Answer from the drawing. Dimensions are ordinates in mm from the lowest x, y and z of the part. A direction names the side the tool comes from. Coordinates: 2 decimals unless noted, no trailing zeros. Order: outer loops, then holes, each group sorted by start corner. A loop starts at its lowest first (then second) coordinate and runs counter-clockwise, first axis right, second up. Notation, with made-up numbers: (36.25, -7.5) -> (84.25, -7.5) arc R19 cw to (84.25, -0.5) -> close; hole circle Ø10 at (1.5, -24.75). An arc over 180 degrees is marked (long way). Answer in a Markdown table with one row per item.
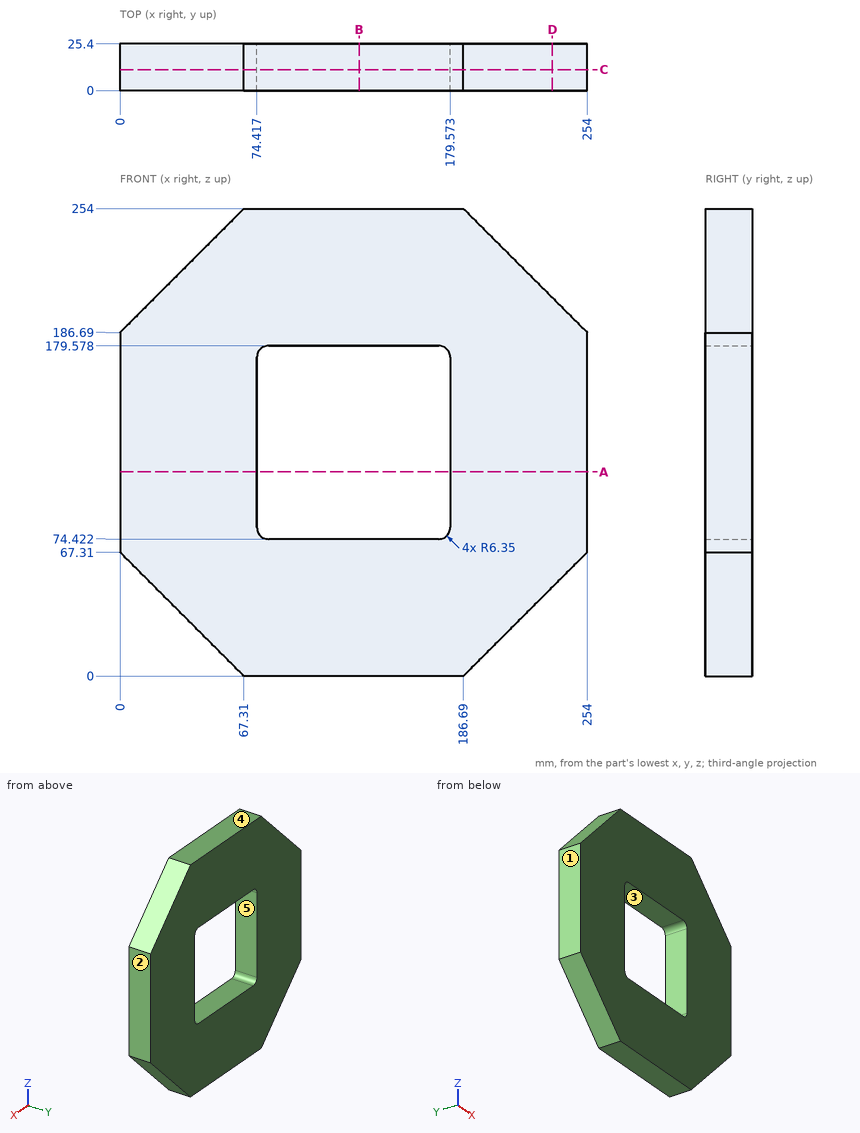
Q1. Consider line 1 (X direction, y = 9.75, z = 133); line 2 (Z direction, x = 122.5, y = 3.5); line 3 (Z direction, x = 177, y = 23). Determine where each line is inside the solid, lowest interval first.
Outcome:
| item | result |
|---|---|
| line 1 | 0 to 74.42, 179.57 to 254 |
| line 2 | 0 to 74.42, 179.58 to 254 |
| line 3 | 0 to 75.67, 178.33 to 254 |
Q2. For the marked faces 4 and 5, determine the directions among +Z, -Z, +X, -X, +Y, -Y from which every point of the face is accessible in a straight line to the end or side of a thin tool.
Outcome:
| item | result |
|---|---|
| face 4 | +Z, +X, -X, +Y, -Y |
| face 5 | +Y, -Y |
Q3. The part is cut by section B-B (x = 130). Write down the section's boundary in (y, z), then the cut area to 3 significant figures.
Outcome:
| item | result |
|---|---|
| outline | (0, 0) -> (25.4, 0) -> (25.4, 74.42) -> (0, 74.42) -> close; (0, 179.58) -> (25.4, 179.58) -> (25.4, 254) -> (0, 254) -> close |
| area | 3,780 mm² |
Q4. The part is cut by section A-A (z = 111). Write down the section's boundary in (x, y).
Outcome:
| item | result |
|---|---|
| outline | (0, 0) -> (74.42, 0) -> (74.42, 25.4) -> (0, 25.4) -> close; (179.57, 0) -> (254, 0) -> (254, 25.4) -> (179.57, 25.4) -> close |
Q5. For a pull along X with two mould halves and no side action, classify the marked faces 1, 2 and 3 as pulls with the +X half, pulls with the -X half, needs draft (parallel to the pull), parting line crosses it, or undercut.
Outcome:
| item | result |
|---|---|
| face 1 | pulls with the -X half |
| face 2 | pulls with the +X half |
| face 3 | undercut |
Q6. The part is cut by section D-D (x = 235). Write down the section's boundary in (y, z), then the cut area to 3 significant figures.
Outcome:
| item | result |
|---|---|
| outline | (0, 48.31) -> (25.4, 48.31) -> (25.4, 205.69) -> (0, 205.69) -> close |
| area | 4,000 mm² |
Q7. The part is cut by section C-C (y = 11.5). Write down the section's boundary in (x, z).
Outcome:
| item | result |
|---|---|
| outline | (0, 67.31) -> (67.31, 0) -> (186.69, 0) -> (254, 67.31) -> (254, 186.69) -> (186.69, 254) -> (67.31, 254) -> (0, 186.69) -> close; hole (74.42, 80.77) arc R6.35 ccw to (80.77, 74.42) -> (173.22, 74.42) arc R6.35 ccw to (179.57, 80.77) -> (179.57, 173.23) arc R6.35 ccw to (173.22, 179.58) -> (80.77, 179.58) arc R6.35 ccw to (74.42, 173.23) -> close |
Q8. Given pin 1 (8 mm diameter, centred on y = 13.5, z = 228.5, fed in from -X); pin 2 (3 mm diameter, centred on x = 220, y = 13, fed in from -Z); pin 3 (8 mm diameter, centred on y = 6, z = 54.5, fed in from -X), each flat-ended and moving along its own axis, determine where each tip first touches the part or whether it passes through.
Outcome:
| item | result |
|---|---|
| pin 1 | x = 37.81 |
| pin 2 | z = 31.81 |
| pin 3 | x = 8.81 |
